Verification items for the finished model (mm, model axes). Face numbers are marked on the shaded views. A direction names the side the tool comes from. Give positions to 0.01 mm unless a question says otherwise; leave off trailing zeros. Loops run counter-clockwise (first coordinate to the right, second up) from the corner with the lowest first, then second, coordinate; pieces in that order, holes last. Notation, with made-up numbers: M 62.25,58 L 84.25,58 A37 ccw 84.25,97 Z; hole C -12,70 d2. An arc over 180 degrees is marked long. Use a Markdown table: item, result.
from build123d import *

# Parameters (mm, degrees)
SKETCH019_R   = 6.25
PAD007_DEPTH  = 10
SKETCH020_R   = 12.5
PAD008_DEPTH  = 5
SKETCH021_R   = 5.2
PAD009_DEPTH  = 0.9
SKETCH022_R   = 2.5
HOLE006_DEPTH = 25


with BuildPart() as part:
    # Sketch019 → Pad007 (new body)
    with BuildSketch(Plane.XY):
        Circle(SKETCH019_R)
    extrude(amount=PAD007_DEPTH)

    # Sketch020 (on Face3 of Pad007) → Pad008 (join)
    with BuildSketch(Plane.XY.offset(10)):
        Circle(SKETCH020_R)
    extrude(amount=PAD008_DEPTH)

    # Sketch021 (on Face3 of Pad008) → Pad009 (join)
    with BuildSketch(Plane.XY.offset(15)):
        Circle(SKETCH021_R)
    extrude(amount=PAD009_DEPTH)

    # Sketch022 (on Face7 of Pad009) → Hole006 (cut)
    with BuildSketch(Plane.XY.offset(15.9)):
        Circle(SKETCH022_R)
    extrude(amount=-HOLE006_DEPTH, mode=Mode.SUBTRACT)


solid = part.part
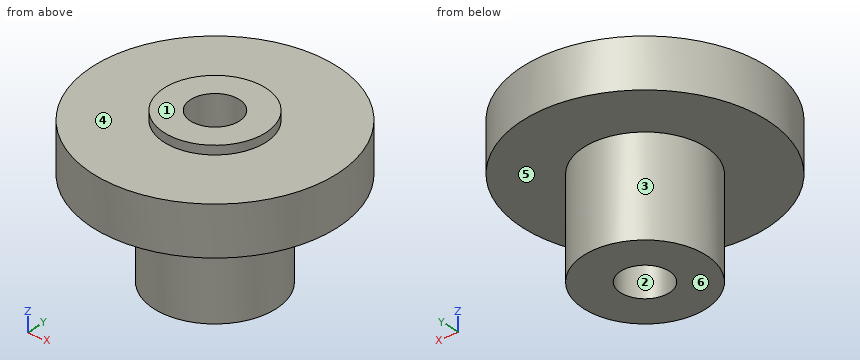
(1) Gauge pin test, flat ends, axial feed: P1, Ø3, axis at x = 8.5, z = 10.5, coming from the +Y side; P2, Ø3, axis at x = -9.5, y = 5, coming from the +Z side; P3, Ø5, axis at y = -8, z = 2.5, coming from the -X side. Record the tip position at first contact, or that the pin passes through.
Results below:
| item | result |
|---|---|
| P1 | y = 10.36 |
| P2 | z = 15 |
| P3 | x = -2.97 |
(2) Material ranges on line 1 (Y direction, x = 0, z = 5); line 2 (Y direction, x = 0, z = 10.25); line 3 (X direction, y = -0.5, z = 3.25), recorded low to high.
Results below:
| item | result |
|---|---|
| line 1 | -6.25 to -2.5, 2.5 to 6.25 |
| line 2 | -12.5 to -2.5, 2.5 to 12.5 |
| line 3 | -6.23 to -2.45, 2.45 to 6.23 |
(3) Cross-section at D-D on y = -4.5. Record the cut outline in (x, z), then the cut area to 3 significant figures.
Results below:
| item | result |
|---|---|
| outline | M -11.66,10 L -4.34,10 L -4.34,0 L 4.34,0 L 4.34,10 L 11.66,10 L 11.66,15 L 2.61,15 L 2.61,15.9 L -2.61,15.9 L -2.61,15 L -11.66,15 Z |
| area | 208 mm^2 |
(4) Cross-section at C-C on z = 6.5. Record the cut outline in (x, y), then the cut area to 3 significant figures.
Results below:
| item | result |
|---|---|
| outline | C 0,0 d12.5; hole C 0,0 d5 |
| area | 103 mm^2 |
(5) Cross-section at A-A on y = 0. Record the cut outline in (x, z), then the cut area to 3 significant figures.
Results below:
| item | result |
|---|---|
| outline | M -12.5,10 L -6.25,10 L -6.25,0 L -2.5,0 L -2.5,15.9 L -5.2,15.9 L -5.2,15 L -12.5,15 Z; M 2.5,0 L 6.25,0 L 6.25,10 L 12.5,10 L 12.5,15 L 5.2,15 L 5.2,15.9 L 2.5,15.9 Z |
| area | 180 mm^2 |
(6) Draft check along X on the marked faces 1, 2 and 3. Enter one of: +X half, -X half, draft (parallel to the pull), parting line (faces both ways), or undercut.
Results below:
| item | result |
|---|---|
| face 1 | draft |
| face 2 | undercut |
| face 3 | parting line |
(7) Set-up check for the marked faces 4, 5 and 6: record each of +Z, -Z, +X, -X, +Y, -Y from which the full face is reachable in a straight line by a thin tool's end or side.
Results below:
| item | result |
|---|---|
| face 4 | +Z |
| face 5 | -Z |
| face 6 | -Z, +X, -X, +Y, -Y |
